from build123d import *

# Parameters (mm, degrees)
PROFILE_EXTRUDE_DEPTH = 170
PROFILE_SHELL_T       = -2
SUPPORT_EXTRUDE_REACH = 182.312
SUPPORT_SKETCH_W      = 2
SUPPORT_SKETCH_H      = 81


with BuildPart() as part:
    # Profile Sketch → Profile Extrude (new body)
    with BuildSketch(Plane(origin=(0, 0, 0), x_dir=(0, 0, -1), z_dir=(1, 0, 0))):
        with BuildLine():
            Line((0, 42.5), (0, -42.5))
            ThreePointArc((0, -42.5), (42.5, 0), (0, 42.5))
        make_face()
    extrude(amount=-PROFILE_EXTRUDE_DEPTH)

    # Profile Shell
    profile_shell_openings = [part.faces().sort_by_distance(p)[0] for p in [
        (-85, 0, 0),
    ]]
    offset(amount=PROFILE_SHELL_T, openings=profile_shell_openings)

    # Support Sketch → Support Extrude (add, up to next)
    with BuildSketch(Plane.XY, mode=Mode.PRIVATE) as support_extrude_sk1:
        with Locations((-127, 0)):
            Rectangle(SUPPORT_SKETCH_W, SUPPORT_SKETCH_H)
    support_extrude_tool1 = extrude(support_extrude_sk1.sketch, amount=-SUPPORT_EXTRUDE_REACH, mode=Mode.PRIVATE) - part.part
    # Support Sketch → Support Extrude (add, up to next)
    with BuildSketch(Plane.XY, mode=Mode.PRIVATE) as support_extrude_sk2:
        with Locations((-43, 0)):
            Rectangle(SUPPORT_SKETCH_W, SUPPORT_SKETCH_H)
    support_extrude_tool2 = extrude(support_extrude_sk2.sketch, amount=-SUPPORT_EXTRUDE_REACH, mode=Mode.PRIVATE) - part.part
    add(support_extrude_tool1.solids().sort_by_distance((-127, 0, 0))[0])
    add(support_extrude_tool2.solids().sort_by_distance((-43, 0, 0))[0])


solid = part.part
Verification items for the finished model (mm, model axes). A direction names the side the tool comes from. Give positions to 0.01 mm unless a question says otherwise; leave off trailing zeros. Loops run counter-clockwise (first coordinate to the right, second up) from the corner with the lowest first, then second, coordinate; pieces in that order, holes last.
1. Go/stop test with flat-tipped pins: P1, Ø1, axis at y = 30, z = -32.5, coming from the -X side (1 decimal); P2, Ø5, axis at x = -64, z = -23, coming from the -Y side; P3, Ø6, axis at x = -131.5, z = -37.5, coming from the -Y side; P4, Ø1, axis at x = -65.5, z = -33, coming from the -Y side. Record where each tip stops, or that it passes through.
Derived:
P1: passes through
P2: stops at y = -37.23
P3: stops at y = -24.82
P4: stops at y = -27.39
2. Tool access check on faces 5 (the flat face through (-44, -1, -15)), 6 (the flat face through (-85, 41, 0)). Record the directions out of +Z, -Z, +X, -X, +Y, -Y that give a thin tool (end or side, any length) a straight path to the whole face; none if there is none.
Derived:
face 5: +Z
face 6: +Z, +X, -X, +Y, -Y
3. Cross-section at B-B on y = 0. Record the cut outline in (x, z), and give its area (3 significant figures).
Derived:
outline: (-170, -42.5) - (0, -42.5) - (0, 0) - (-2, 0) - (-2, -40.5) - (-42, -40.5) - (-42, 0) - (-44, 0) - (-44, -40.5) - (-126, -40.5) - (-126, 0) - (-128, 0) - (-128, -40.5) - (-168, -40.5) - (-168, 0) - (-170, 0) - close
area: 664 mm2
4. Cross-section at C-C on x = -114. Record the cut outline in (y, z), and give its area (3 significant figures).
Derived:
outline: (-42.5, 0) arc R42.5 ccw to (42.5, 0) - (40.5, 0) arc R40.5 cw to (-40.5, 0) - close
area: 261 mm2
5. Release check for a two-part mould opening along X. For faces 1 (the flat face through (-128, -1, -15)), 2 (the flat face through (0, 1, -16)), 3 (the cylindrical face through (-83.81, -0.93, -42.49)), 4 (the flat face through (-170, 1, -16)) record: +X half, -X half, draft (parallel to the pull), parting line (faces both ways), or undercut.
Derived:
face 1: undercut
face 2: +X half
face 3: draft
face 4: -X half
6. Cross-section at A-A on z = -8. Record the cut outline in (x, y).
Derived:
outline: (-170, -41.74) - (0, -41.74) - (0, 41.74) - (-170, 41.74) - close; hole (-168, -39.7) - (-128, -39.7) - (-128, 39.7) - (-168, 39.7) - close; hole (-126, -39.7) - (-44, -39.7) - (-44, 39.7) - (-126, 39.7) - close; hole (-42, -39.7) - (-2, -39.7) - (-2, 39.7) - (-42, 39.7) - close
7. Cross-section at D-D on z = -32. Record the cut outline in (x, y).
Derived:
outline: (-170, -27.97) - (0, -27.97) - (0, 27.97) - (-170, 27.97) - close; hole (-168, -24.82) - (-128, -24.82) - (-128, 24.82) - (-168, 24.82) - close; hole (-126, -24.82) - (-44, -24.82) - (-44, 24.82) - (-126, 24.82) - close; hole (-42, -24.82) - (-2, -24.82) - (-2, 24.82) - (-42, 24.82) - close
8. Material ranges on probe 1 along X at (y, z) = (15, -30); probe 2 along Y at (x, z) = (-145, -23); probe 3 along Y at (x, z) = (-97, -20), recorded low to high.
Derived:
probe 1: x = -170 to -168, -128 to -126, -44 to -42, -2 to 0
probe 2: y = -35.74 to -33.34, 33.34 to 35.74
probe 3: y = -37.5 to -35.22, 35.22 to 37.5
